```python
from build123d import *

# Parameters (mm, degrees)
STOCK_MODIFYCOMPONENTPART_1_START = 6
STOCK_MODIFYCOMPONENTPART_1_DEPTH = 0.6
SKETCH1_W                         = 3
SKETCH1_H                         = 1.6
BOSS_EXTRUDE1_DEPTH               = 1


# Read off the part's stored shape, not the designer's step: Stock-ModifyComponentPart-1
with BuildPart() as part:
    # Stock-ModifyComponentPart-1 outline → Stock-ModifyComponentPart-1 (new body)
    with BuildSketch(Plane(origin=(0, 0, 0), x_dir=(1, 0, 0), z_dir=(0, 1, 0)).offset(STOCK_MODIFYCOMPONENTPART_1_START)):
        with BuildLine():
            Line((12.25, 3.3), (12.25, 7))
            ThreePointArc((12.25, 7), (11.664213562, 8.414213562), (10.25, 9))
            Line((10.25, 9), (-10.25, 9))
            ThreePointArc((-10.25, 9), (-11.664213562, 8.414213562), (-12.25, 7))
            Line((-12.25, 7), (-12.25, 3.3))
            Line((-12.25, 3.3), (-21.75, 3.3))
            Line((-21.75, 3.3), (-21.75, -3.3))
            Line((-21.75, -3.3), (-12.25, -3.3))
            Line((-12.25, -3.3), (-12.25, -7))
            ThreePointArc((-12.25, -7), (-11.664213562, -8.414213562), (-10.25, -9))
            Line((-10.25, -9), (10.25, -9))
            ThreePointArc((10.25, -9), (11.664213562, -8.414213562), (12.25, -7))
            Line((12.25, -7), (12.25, -3.3))
            Line((12.25, -3.3), (21.75, -3.3))
            Line((21.75, -3.3), (21.75, 3.3))
            Line((21.75, 3.3), (12.25, 3.3))
        make_face()
    extrude(amount=STOCK_MODIFYCOMPONENTPART_1_DEPTH)

    # Sketch1 → Boss-Extrude1 (add)
    with BuildSketch(Plane(origin=(0, 6.6, 0), x_dir=(1, 0, 0), z_dir=(0, 1, 0))):
        Rectangle(SKETCH1_W, SKETCH1_H)
    extrude(amount=BOSS_EXTRUDE1_DEPTH)


solid = part.part
```
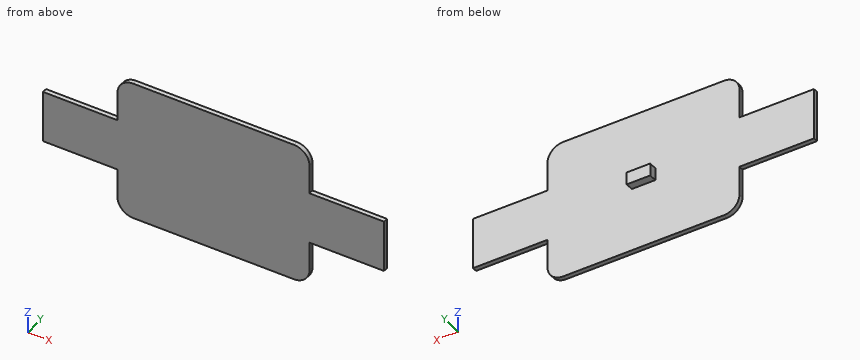
Can you work these out from the model? Positions are in its coordinate system, mm. Coordinates: 2 decimals unless noted, no trailing zeros. Loops run counter-clockwise (first coordinate to the right, second up) from the corner with the lowest first, then second, coordinate; pieces in that order, holes last. Notation, with made-up numbers: M 87,18.25 L 132,18.25 A6 ccw 132,24.25 Z; hole C -18.75,18.5 d2. An arc over 180 degrees is marked long. Put each result on its own line as item: value. Start each with the question number.
(1) Imagine slicing it at D-D on x = 6. List the corners of the cut face in (y, z) for me, and give its area (3 significant figures).
(2) I need wall thicknesses on probe 1 along Z at (x, y) = (-13, 6.35); probe 2 along Y at (x, z) = (-2.5, -4); probe 3 along Z at (x, y) = (-0.5, 7.45). Which ranges of each line are inside material? Lowest first, please.
(3) Imagine slicing it at B-B on y = 6.3. List the corners of the cut face in (x, z) for me.
(4) Imagine slicing it at A-A on x = -1. List the corners of the cut face in (y, z) for me.
(5) Will these pins go through, and if not, where does the flat tip stop? pin 1 Ø0.5 at (y, z) = (6.5, 6) entering from +X; pin 2 Ø1.5 at (x, z) = (-4.5, 4) entering from +Y; pin 3 Ø0.5 at (x, y) = (-14.5, 6.5) entering from +Z.
(6) Imagine slicing it at C-C on z = 3.75. List the corners of the cut face in (x, y) for me, and give its area (3 significant figures).
Worked answers:
1. outline: M 6,-9 L 6.6,-9 L 6.6,9 L 6,9 Z
1. area: 10.8 mm2
2. probe 1: z = -3.3 to 3.3
2. probe 2: y = 6 to 6.6
2. probe 3: z = -0.8 to 0.8
3. outline: M -21.75,-3.3 L -12.25,-3.3 L -12.25,-7 A2 ccw -10.25,-9 L 10.25,-9 A2 ccw 12.25,-7 L 12.25,-3.3 L 21.75,-3.3 L 21.75,3.3 L 12.25,3.3 L 12.25,7 A2 ccw 10.25,9 L -10.25,9 A2 ccw -12.25,7 L -12.25,3.3 L -21.75,3.3 Z
4. outline: M 6,-9 L 6.6,-9 L 6.6,-0.8 L 7.6,-0.8 L 7.6,0.8 L 6.6,0.8 L 6.6,9 L 6,9 Z
5. pin 1: stops at x = 12.25
5. pin 2: stops at y = 6.6
5. pin 3: stops at z = 3.3
6. outline: M -12.25,6 L 12.25,6 L 12.25,6.6 L -12.25,6.6 Z
6. area: 14.7 mm2
